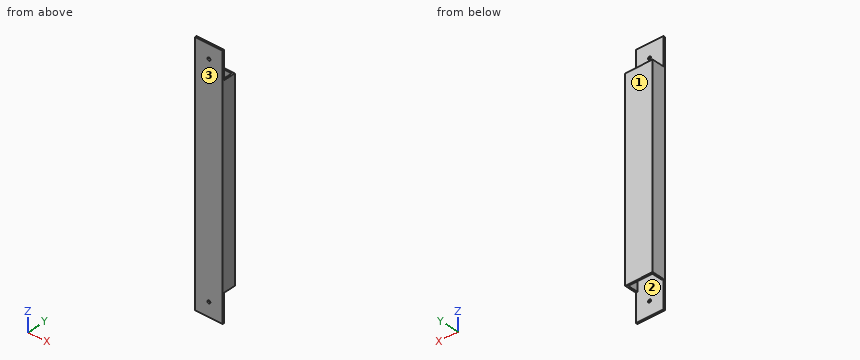
from build123d import *

# Parameters (mm, degrees)
SKETCH1_W           = 50.8
SKETCH1_H           = 25.4
SKETCH1_W_2         = 44.45
SKETCH1_H_2         = 19.05
BOSS_EXTRUDE1_DEPTH = 457.2
SKETCH2_R           = 2.667
CUT_EXTRUDE1_DEPTH  = 26.4
SKETCH3_W           = 50.8
SKETCH3_H           = 50.8
CUT_EXTRUDE2_DEPTH  = 22.225


with BuildPart() as part:
    # Sketch1 → Boss-Extrude1 (new body)
    with BuildSketch(Plane.XY):
        Rectangle(SKETCH1_W, SKETCH1_H)
        Rectangle(SKETCH1_W_2, SKETCH1_H_2, mode=Mode.SUBTRACT)
    extrude(amount=BOSS_EXTRUDE1_DEPTH)

    # Sketch2 → Cut-Extrude1 (cut, through all)
    with BuildSketch(Plane(origin=(0, 12.7, 0), x_dir=(1, 0, 0), z_dir=(0, 1, 0))):
        with Locations((0, -431.8)):
            Circle(SKETCH2_R)
        with Locations((0, -25.4)):
            Circle(SKETCH2_R)
    extrude(amount=-CUT_EXTRUDE1_DEPTH, mode=Mode.SUBTRACT)

    # Sketch3 → Cut-Extrude2 (cut)
    with BuildSketch(Plane(origin=(0, 12.7, 0), x_dir=(1, 0, 0), z_dir=(0, 1, 0))):
        with Locations((0, -431.8)):
            Rectangle(SKETCH3_W, SKETCH3_H)
        with Locations((0, -25.4)):
            Rectangle(SKETCH3_W, SKETCH3_H)
    extrude(amount=-CUT_EXTRUDE2_DEPTH, mode=Mode.SUBTRACT)


solid = part.part
The listing builds one solid part. Answer for the finished solid, in the listing's coordinates (mm). Face numbers are marked on the shaded views. Round coordinates to 2 decimals unless told otherwise and drop trailing zeros. Order: outer loops, then holes, each group sorted by start corner. A loop starts at its lowest first (then second) coordinate and runs counter-clockwise, first axis right, second up. Notation, with made-up numbers: M 1.25,-6.75 L 14.25,-6.75 A16 ccw 14.25,5.25 Z; hole C 36,74 d8. An arc over 180 degrees is marked long. Answer in a Markdown table with one row per item. Add a question column.
1) Consider line 1 along Z through (x, y) = (0, -10.75); line 2 along X through (y, z) = (4.25, 374) (3 decimals); line 3 along Y through (x, z) = (-15, 118.5) (3 decimals). Determine where each line is inside the solid, lowest interval first. Write a range as from..to.
2) Determine the mould class of the marked faces 1, 2 and 3 for opening direction Y: pulls with the +Y half, pulls with the -Y half, needs draft (parallel to the pull), parting line crosses it, or undercut.
3) The part is cut by section D-D on z = 37. Determine the outline of the cut face in (x, y) (3 decimals).
4) Flat-ended cylindrical pins translate along their axes: pin 1 Ø6 at (x, y) = (5, 8.5) entering from -Z; pin 2 Ø6 at (x, z) = (0, 431.8) entering from +Y (3 decimals). Find the tip coordinate at first contact, or state that the pin passes through.
5) The part is cut by section B-B on y = 1.5. Determine the outline of the cut face in (x, z) (3 decimals), plus the area to 3 significant figures.
6) The part is cut by section C-C on z = 253. Determine the outline of the cut face in (x, y) (3 decimals).
7) The part is cut by section A-A on x = -13.5. Determine the outline of the cut face in (y, z) (3 decimals).
Findings below:
| question | item | result |
|---|---|---|
| 1 | line 1 | z = 0..22.73, 28.07..429.13, 434.47..457.2 |
| 1 | line 2 | x = -25.4..-22.225, 22.225..25.4 |
| 1 | line 3 | y = -12.7..-9.525, 9.525..12.7 |
| 2 | face 1 | pulls with the +Y half |
| 2 | face 2 | undercut |
| 2 | face 3 | pulls with the -Y half |
| 3 | outline | M -25.4,-12.7 L 25.4,-12.7 L 25.4,-9.525 L -25.4,-9.525 Z |
| 4 | pin 1 | stops at z = 50.8 |
| 4 | pin 2 | stops at y = -9.525 |
| 5 | outline | M -25.4,50.8 L -22.225,50.8 L -22.225,406.4 L -25.4,406.4 Z; M 22.225,50.8 L 25.4,50.8 L 25.4,406.4 L 22.225,406.4 Z |
| 5 | area | 2,260 mm² |
| 6 | outline | M -25.4,-12.7 L 25.4,-12.7 L 25.4,12.7 L -25.4,12.7 Z; hole M -22.225,-9.525 L 22.225,-9.525 L 22.225,9.525 L -22.225,9.525 Z |
| 7 | outline | M -12.7,0 L -9.525,0 L -9.525,457.2 L -12.7,457.2 Z; M 9.525,50.8 L 12.7,50.8 L 12.7,406.4 L 9.525,406.4 Z |
